```python
from build123d import *

# Parameters (mm, degrees)
ESQUISSE1_W                = 203.2
ESQUISSE1_H                = 203.2
BOSS_EXTRU_1_DEPTH         = 6.35
ESQUISSE2_R                = 3.925
ENL_V_MAT_EXTRU_1_DEPTH    = 144.824345992
ESQUISSE5_R                = 2.6
ENL_V_MAT_EXTRU_4_DEPTH    = 144.824345992
ESQUISSE6_R                = 2.5
ENL_V_MAT_EXTRU_5_DEPTH    = 144.824345992
ESQUISSE7_R                = 2.5
ENL_V_MAT_EXTRU_6_DEPTH    = 144.824345992
ESQUISSE8_R                = 4
ENL_V_MAT_EXTRU_7_DEPTH    = 144.824345992
ESQUISSE9_R                = 2.5
ENL_V_MAT_EXTRU_8_DEPTH    = 144.824345992
SYM_TRIE2_COPY_1_SKETCH_R  = 2.5
SYM_TRIE2_COPY_1_DEPTH     = 144.824345992
ENL_V_MAT_EXTRU_9_DEPTH    = 144.824345992
CONG_1_R                   = 4
ENL_V_MAT_EXTRU_10_DEPTH   = 144.824345992
R_P_TITION_LIN_AIRE3_COUNT = 2
R_P_TITION_LIN_AIRE3_PITCH = 86


with BuildPart() as part:
    # Esquisse1 → Boss.-Extru.1 (new body)
    with BuildSketch(Plane(origin=(0, 0, 0), x_dir=(1, 0, 0), z_dir=(0, 1, 0))):
        Rectangle(ESQUISSE1_W, ESQUISSE1_H)
    extrude(amount=BOSS_EXTRU_1_DEPTH)

    # Esquisse2 → Enlèv. mat.-Extru.1 (cut, through all)
    with BuildSketch(Plane(origin=(0, 6.35, 0), x_dir=(1, 0, 0), z_dir=(0, 1, 0))):
        with Locations(Location((-75, 65, 0), (0, 0, 270))):
            Circle(ESQUISSE2_R)
        with Locations(Location((75, 65, 0), (0, 0, 270))):
            Circle(ESQUISSE2_R)
        with Locations(Location((0, -65, 0), (0, 0, 270))):
            Circle(ESQUISSE2_R)
    extrude(amount=-ENL_V_MAT_EXTRU_1_DEPTH, mode=Mode.SUBTRACT)

    # Esquisse5 → Enlèv. mat.-Extru.4 (cut, through all)
    with BuildSketch(Plane(origin=(0, 6.35, 0), x_dir=(1, 0, 0), z_dir=(0, 1, 0))):
        with Locations(Location((-35.9, 49.85, 0), (0, 0, 270))):
            Circle(ESQUISSE5_R)
        with Locations(Location((-35.9, 79.85, 0), (0, 0, 270))):
            Circle(ESQUISSE5_R)
        with Locations(Location((35.6, 49.85, 0), (0, 0, 270))):
            Circle(ESQUISSE5_R)
        with Locations(Location((35.6, 79.85, 0), (0, 0, 270))):
            Circle(ESQUISSE5_R)
    enl_v_mat_extru_4 = extrude(amount=-ENL_V_MAT_EXTRU_4_DEPTH, mode=Mode.SUBTRACT)

    # Esquisse6 → Enlèv. mat.-Extru.5 (cut, through all)
    with BuildSketch(Plane(origin=(0, 6.35, 0), x_dir=(1, 0, 0), z_dir=(0, 1, 0))):
        with Locations(Location((93.6, -93.6, 0), (0, 0, 270))):
            Circle(ESQUISSE6_R)
        with Locations(Location((-93.6, -93.6, 0), (0, 0, 270))):
            Circle(ESQUISSE6_R)
        with Locations(Location((-93.6, 93.6, 0), (0, 0, 270))):
            Circle(ESQUISSE6_R)
        with Locations(Location((93.6, 93.6, 0), (0, 0, 270))):
            Circle(ESQUISSE6_R)
    extrude(amount=-ENL_V_MAT_EXTRU_5_DEPTH, mode=Mode.SUBTRACT)

    # Esquisse7 → Enlèv. mat.-Extru.6 (cut, through all)
    with BuildSketch(Plane(origin=(0, 6.35, 0), x_dir=(1, 0, 0), z_dir=(0, 1, 0))):
        with Locations(Location((15.588457268, -56, 0), (0, 0, 270))):
            Circle(ESQUISSE7_R)
        with Locations(Location((-15.588457268, -56, 0), (0, 0, 270))):
            Circle(ESQUISSE7_R)
        with Locations(Location((0, -83, 0), (0, 0, 270))):
            Circle(ESQUISSE7_R)
        with Locations(Location((90.588457268, 56, 0), (0, 0, 270))):
            Circle(ESQUISSE7_R)
        with Locations(Location((59.411542732, 56, 0), (0, 0, 270))):
            Circle(ESQUISSE7_R)
        with Locations(Location((75, 83, 0), (0, 0, 270))):
            Circle(ESQUISSE7_R)
        with Locations(Location((-90.589923123, 55.999154304, 0), (0, 0, 270))):
            Circle(ESQUISSE7_R)
        with Locations(Location((-59.413008586, 55.999154304, 0), (0, 0, 270))):
            Circle(ESQUISSE7_R)
        with Locations(Location((-75.001465855, 82.999154304, 0), (0, 0, 270))):
            Circle(ESQUISSE7_R)
    extrude(amount=-ENL_V_MAT_EXTRU_6_DEPTH, mode=Mode.SUBTRACT)

    # Esquisse8 → Enlèv. mat.-Extru.7 (cut, through all)
    with BuildSketch(Plane(origin=(0, 6.35, 0), x_dir=(1, 0, 0), z_dir=(0, 1, 0))):
        with Locations(Location((0, 10.325, 0), (0, 0, 270))):
            Circle(ESQUISSE8_R)
    extrude(amount=-ENL_V_MAT_EXTRU_7_DEPTH, mode=Mode.SUBTRACT)

    # Esquisse9 → Enlèv. mat.-Extru.8 (cut, through all)
    with BuildSketch(Plane.XZ):
        with Locations(Location((56, -85, 0), (0, 0, 270))):
            Circle(ESQUISSE9_R)
        with Locations(Location((82, 0, 0), (0, 0, 270))):
            Circle(ESQUISSE9_R)
    enl_v_mat_extru_8 = extrude(amount=-ENL_V_MAT_EXTRU_8_DEPTH, mode=Mode.SUBTRACT)

    # Symétrie1: Enlèv. mat.-Extru.8 across plane
    add(enl_v_mat_extru_8.mirror(Plane.XY), mode=Mode.SUBTRACT)

    # Symétrie2: Enlèv. mat.-Extru.8 across plane
    add(enl_v_mat_extru_8.mirror(Plane(origin=(0, 0, 0), x_dir=(0, 0, 1), z_dir=(1, 0, 0))), mode=Mode.SUBTRACT)

    # Symétrie2 copy 1 sketch → Symétrie2 copy 1 (cut, through all)
    with BuildSketch(Plane(origin=(0, 0, 0), x_dir=(-1, 0, 0), z_dir=(0, -1, 0))):
        with Locations(Location((56, -85, 0), (0, 0, 270))):
            Circle(SYM_TRIE2_COPY_1_SKETCH_R)
        with Locations(Location((82, 0, 0), (0, 0, 270))):
            Circle(SYM_TRIE2_COPY_1_SKETCH_R)
    extrude(amount=-SYM_TRIE2_COPY_1_DEPTH, mode=Mode.SUBTRACT)

    # Esquisse11 → Enlèv. mat.-Extru.9 (cut, through all)
    with BuildSketch(Plane.XZ):
        Polygon((-60.5033321, -85), (-58.25166605, -88.9), (-53.74833395, -88.9), (-51.4966679, -85), (-53.74833395, -81.1), (-58.25166605, -81.1), align=None)
        Polygon((-86.5033321, 0), (-84.25166605, -3.9), (-79.74833395, -3.9), (-77.4966679, 0), (-79.74833395, 3.9), (-84.25166605, 3.9), align=None)
        Polygon((-60.5033321, 85), (-58.25166605, 81.1), (-53.74833395, 81.1), (-51.4966679, 85), (-53.74833395, 88.9), (-58.25166605, 88.9), align=None)
        Polygon((51.4966679, 85), (53.74833395, 81.1), (58.25166605, 81.1), (60.5033321, 85), (58.25166605, 88.9), (53.74833395, 88.9), align=None)
        Polygon((77.4966679, 0), (79.74833395, -3.9), (84.25166605, -3.9), (86.5033321, 0), (84.25166605, 3.9), (79.74833395, 3.9), align=None)
        Polygon((60.5033321, -85), (58.25166605, -81.1), (53.74833395, -81.1), (51.4966679, -85), (53.74833395, -88.9), (58.25166605, -88.9), align=None)
    extrude(amount=-ENL_V_MAT_EXTRU_9_DEPTH, mode=Mode.SUBTRACT)

    # Congé1
    cong_1_edges = [part.edges().sort_by_distance(p)[0] for p in [
        (101.6, 3.175, 101.6),
        (-101.6, 3.175, 101.6),
        (-101.6, 3.175, -101.6),
        (101.6, 3.175, -101.6),
    ]]
    fillet(cong_1_edges, radius=CONG_1_R)

    # Esquisse13 → Enlèv. mat.-Extru.10 (cut, through all)
    with BuildSketch(Plane(origin=(0, 6.35, 0), x_dir=(1, 0, 0), z_dir=(0, 1, 0))):
        Polygon((-16.978069991, 0.149999997), (16.978069991, 0.149999997), (21.15, -4.021930012), (21.15, -37.978069994), (16.978069991, -42.150000003), (-16.978069991, -42.150000003), (-21.15, -37.978069994), (-21.15, -4.021930012), align=None)
    extrude(amount=-ENL_V_MAT_EXTRU_10_DEPTH, mode=Mode.SUBTRACT)

    # Répétition linéaire3: Enlèv. mat.-Extru.4 ×2
    with Locations(*[(0, 0, i * R_P_TITION_LIN_AIRE3_PITCH) for i in range(1, R_P_TITION_LIN_AIRE3_COUNT)]):
        add(enl_v_mat_extru_4, mode=Mode.SUBTRACT)


solid = part.part
```
Input: part model. Units: mm. Frame: model coordinates. A direction names the side the tool comes from. Coordinates: 2 decimals unless noted, no trailing zeros. Loops run counter-clockwise (first coordinate to the right, second up) from the corner with the lowest first, then second, coordinate; pieces in that order, holes last. Notation, with made-up numbers: (9, 26) -> (53, 26) arc R34 cw to (53, 57) -> close; hole circle Ø10 at (-6, 3). An arc over 180 degrees is marked (long way). Use a Markdown table: item, result.
1) Cut plane B-B (z = 93.6). Return the cut outline in (x, y).
Results found:
| item | result |
|---|---|
| outline | (-101.6, 0) -> (-96.1, 0) -> (-96.1, 6.35) -> (-101.6, 6.35) -> close; (-91.1, 0) -> (91.1, 0) -> (91.1, 6.35) -> (-91.1, 6.35) -> close; (96.1, 0) -> (101.6, 0) -> (101.6, 6.35) -> (96.1, 6.35) -> close |
2) Material intervals for line 1 along X through (y, z) = (3.75, -79.85); line 2 along X through (y, z) = (4.5, 56); line 3 along X through (y, z) = (2.5, -10.5), sorted ascending. Write a range as from..to.
Results found:
| item | result |
|---|---|
| line 1 | x = -101.6..-38.5, -33.3..33, 38.2..101.6 |
| line 2 | x = -101.6..-18.09, -13.09..13.09, 18.09..101.6 |
| line 3 | x = -101.6..-4, 4..101.6 |
3) Cut plane A-A (z = -56). Return the cut outline in (x, y).
Results found:
| item | result |
|---|---|
| outline | (-101.6, 0) -> (-93.09, 0) -> (-93.09, 6.35) -> (-101.6, 6.35) -> close; (-88.09, 0) -> (-61.91, 0) -> (-61.91, 6.35) -> (-88.09, 6.35) -> close; (-56.91, 0) -> (56.91, 0) -> (56.91, 6.35) -> (-56.91, 6.35) -> close; (61.91, 0) -> (88.09, 0) -> (88.09, 6.35) -> (61.91, 6.35) -> close; (93.09, 0) -> (101.6, 0) -> (101.6, 6.35) -> (93.09, 6.35) -> close |
4) Cut plane D-D (y = 1.5). Give the number of separate pieces and of enclosed holes in the cut face, then the cut area to 3 significant figures.
Results found:
| item | result |
|---|---|
| separate pieces | 1 |
| enclosed holes | 32 |
| area | 38,600 mm2 |
5) Pull-direction query (X, two-part tool) for faces 1 (the flat face through (-1, 3, 101.6)), 2 (the flat face through (-101.6, 3, 1)), 3 (the cylindrical face through (61.52, 3.22, -54.66)); classes: released by +X, released by -X, zero draft, split by the parting line, or undercut.
Results found:
| item | result |
|---|---|
| face 1 | zero draft |
| face 2 | released by -X |
| face 3 | undercut |
6) Access query for faces 4 (the flat face through (-1, 0, -1)), 5 (the flat face through (0, 3, -0.15)). Directions: +Z, -Z, +X, -X, +Y, -Y. A direction counts if a zero-diameter tool reaches every point of the face in a straight line with its end or side. Return the directions, or none.
Results found:
| item | result |
|---|---|
| face 4 | +Z, -Z, +X, -X, -Y |
| face 5 | +Y, -Y |
7) Cut plane C-C (z = 65). Return the cut outline in (x, y) (3 decimals).
Results found:
| item | result |
|---|---|
| outline | (-101.6, 0) -> (-3.925, 0) -> (-3.925, 6.35) -> (-101.6, 6.35) -> close; (3.925, 0) -> (101.6, 0) -> (101.6, 6.35) -> (3.925, 6.35) -> close |
